Check sheet for the drawn part. Datum: minimum x, y, z corner. Units: mm. A direction names the side the tool comes from. Give positions to 0.01 mm unless a question says otherwise; leave off trailing zeros. Loops run counter-clockwise (first coordinate to the right, second up) from the corner with the lowest first, then second, coordinate; pieces in that order, holes last.
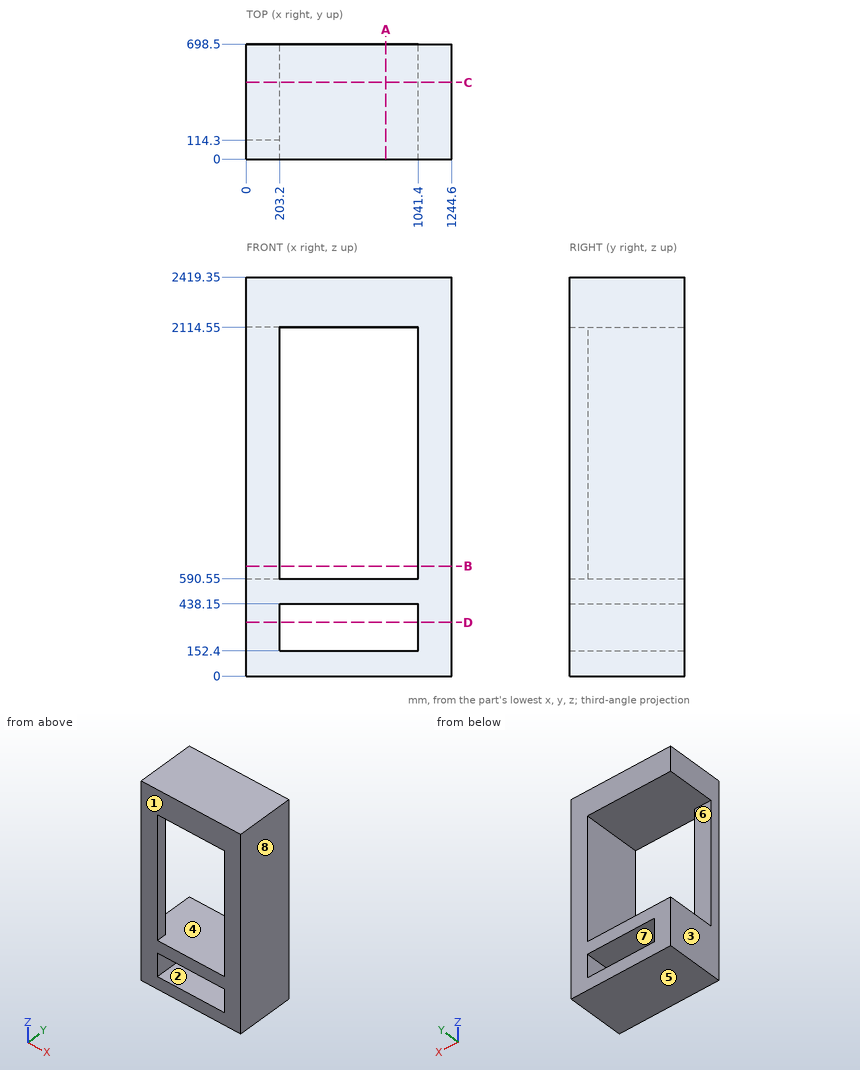
1) Tool access check on the marked faces 4, 5, 6, 7 and 8. Record the directions out of +Z, -Z, +X, -X, +Y, -Y that give a thin tool (end or side, any length) a straight path to the whole face; none if there is none.
2) Scan lines: line 1 along Z through (x, y) = (806, 556); line 2 along X through (y, z) = (51.5, 1117.5); line 3 along X through (y, z) = (366.5, 801.5). Record each from-to range of solid material in increasing order.
3) Sectioned sample at C-C on y = 466. Enter the section's corners in (x, z).
4) Mould release check, pull along X, two halves, no side actions. Record for the marked faces 1, 2 and 3: +X half, -X half, draft (parallel to the pull), parting line (faces both ways), or undercut.
5) Depth check by flat-ended pin: P1, Ø10, axis at y = 136.5, z = 974.5, coming from the -X side; P2, Ø3, axis at x = 137.5, z = 1062, coming from the +Y side. Enter the tip coordinate at first touch or a pass-through.
6) Sectioned sample at B-B on z = 667. Enter the section's corners in (x, y).
7) Sectioned sample at D-D on z = 326. Enter the section's corners in (x, y), plus the area to 3 significant figures.
8) Sectioned sample at A-A on x = 846.5. Enter the section's corners in (y, z).
Determined:
1. face 4: +Y
1. face 5: -Z, +X, -X, +Y, -Y
1. face 6: -X, +Y
1. face 7: +Y, -Y
1. face 8: +Z, -Z, +X, +Y, -Y
2. line 1: z = 0 to 152.4, 438.15 to 590.55, 2114.55 to 2419.35
2. line 2: x = 0 to 203.2, 1041.4 to 1244.6
2. line 3: x = 1041.4 to 1244.6
3. outline: (0, 0) - (1244.6, 0) - (1244.6, 2419.35) - (0, 2419.35) - (0, 2114.55) - (1041.4, 2114.55) - (1041.4, 590.55) - (0, 590.55) - close; hole (203.2, 152.4) - (1041.4, 152.4) - (1041.4, 438.15) - (203.2, 438.15) - close
4. face 1: draft
4. face 2: undercut
4. face 3: -X half
5. P1: stops at x = 1041.4
5. P2: stops at y = 114.3
6. outline: (0, 0) - (203.2, 0) - (203.2, 114.3) - (0, 114.3) - close; (1041.4, 0) - (1244.6, 0) - (1244.6, 698.5) - (1041.4, 698.5) - close
7. outline: (0, 0) - (203.2, 0) - (203.2, 698.5) - (0, 698.5) - close; (1041.4, 0) - (1244.6, 0) - (1244.6, 698.5) - (1041.4, 698.5) - close
7. area: 284,000 mm2
8. outline: (0, 0) - (698.5, 0) - (698.5, 152.4) - (0, 152.4) - close; (0, 438.15) - (698.5, 438.15) - (698.5, 590.55) - (0, 590.55) - close; (0, 2114.55) - (698.5, 2114.55) - (698.5, 2419.35) - (0, 2419.35) - close
